Build history of the part. All positions in model axes, mm. A direction names the side the tool comes from. Round coordinates to 2 decimals unless told otherwise and drop trailing zeros. Order: outer loops, then holes, each group sorted by start corner. A loop starts at its lowest first (then second) coordinate and runs counter-clockwise, first axis right, second up. Notation, with made-up numbers: M 8,75.5 L 30,75.5 A9 cw 30,89.5 Z; hole C 53.25,29.25 d2. An arc over 180 degrees is marked long. Use CSV: the item, a comma, the result in double quotes.
from build123d import *

# Parameters (mm, degrees)
SKETCH1_W                    = 50
SKETCH1_H                    = 50
BASE_FLANGE2_DEPTH           = 3
EDGE_FLANGE1_STRIP_W         = 16
EDGE_FLANGE1_STRIP_H         = 3
EDGE_FLANGE1_STRIP_CUT_DEPTH = 50
EDGE_FLANGE1_DEPTH           = 50
EDGE_FLANGE1_PROFILE_R       = 6.25
EDGE_FLANGE1_PROFILE_R_2     = 5.5
EDGE_FLANGE1_FLAT_DEPTH      = 3
SKETCH22_R                   = 6.5
CUT_EXTRUDE1_DEPTH           = 10


# Sheet-metal steps are written as plain solids
with BuildPart() as part:
    # Sketch1 → Base-Flange2 (new body)
    with BuildSketch(Plane.XY):
        Rectangle(SKETCH1_W, SKETCH1_H)
    extrude(amount=-BASE_FLANGE2_DEPTH)

    # Edge-Flange1 strip (across the edge) → Edge-Flange1 strip cut (cut)
    with BuildSketch(Plane(origin=(25, -25, 0), x_dir=(-1, 0, 0), z_dir=(0, 1, 0))):
        with Locations((-3, -1.5)):
            Rectangle(EDGE_FLANGE1_STRIP_W, EDGE_FLANGE1_STRIP_H)
    edge_flange1_strip_cut = extrude(amount=EDGE_FLANGE1_STRIP_CUT_DEPTH, mode=Mode.SUBTRACT)

    # Edge-Flange1 bend section (across the edge) → Edge-Flange1 (add)
    with BuildSketch(Plane(origin=(25, -25, 0), x_dir=(-1, 0, 0), z_dir=(0, 1, 0))):
        with BuildLine():
            Line((0, 2), (3, 2))
            ThreePointArc((3, 2), (3.585786438, 0.585786438), (5, 0))
            Line((5, 0), (5, -3))
            ThreePointArc((5, -3), (1.464466094, -1.535533906), (0, 2))
        make_face()
    edge_flange1 = extrude(amount=EDGE_FLANGE1_DEPTH)

    # Edge-Flange1 profile (on flange) → Edge-Flange1 flat (add)
    with BuildSketch(Plane.YZ.offset(25)):
        with BuildLine():
            ThreePointArc((32.731549172, 73.12961498), (30.399526878, 85.843718314), (17.474995057, 85.635802941))
            Line((17.474995057, 85.635802941), (-17.56059029, 55.179833247))
            ThreePointArc((-17.56059029, 55.179833247), (-20.099612709, 51.779669871), (-21, 47.632737445))
            Line((-21, 47.632737445), (-21, 27.69))
            Line((-21, 27.69), (-25, 25.69))
            Line((-25, 25.69), (-25, 2))
            Line((-25, 2), (25, 2))
            Line((25, 2), (25, 25.69))
            Line((25, 25.69), (21, 27.69))
            Line((21, 27.69), (21, 52.19))
            Line((21, 52.19), (32.731549172, 73.12961498))
        make_face()
        with Locations((0, 52.19)):
            Circle(EDGE_FLANGE1_PROFILE_R, mode=Mode.SUBTRACT)
        with Locations((24.06, 78.11)):
            Circle(EDGE_FLANGE1_PROFILE_R_2, mode=Mode.SUBTRACT)
    edge_flange1_flat = extrude(amount=-EDGE_FLANGE1_FLAT_DEPTH)

    # Mirror1: Edge-Flange1 strip cut, Edge-Flange1, Edge-Flange1 flat across plane
    add(edge_flange1_strip_cut.mirror(Plane(origin=(0, 0, 0), x_dir=(0, 0, 1), z_dir=(1, 0, 0))), mode=Mode.SUBTRACT)
    add(edge_flange1.mirror(Plane(origin=(0, 0, 0), x_dir=(0, 0, 1), z_dir=(1, 0, 0))))
    add(edge_flange1_flat.mirror(Plane(origin=(0, 0, 0), x_dir=(0, 0, 1), z_dir=(1, 0, 0))))

    # Sketch22 → Cut-Extrude1 (cut)
    with BuildSketch(Plane(origin=(0, 0, -3), x_dir=(-1, 0, 0), z_dir=(0, 0, -1))):
        Circle(SKETCH22_R)
    extrude(amount=-CUT_EXTRUDE1_DEPTH, mode=Mode.SUBTRACT)


solid = part.part
(1) Cut at A-A, the plane x = 0. Give the cut face in (y, z), and give its area (3 significant figures).
Answer block:
outline,"M -25,-3 L -6.5,-3 L -6.5,0 L -25,0 Z; M 6.5,-3 L 25,-3 L 25,0 L 6.5,0 Z"
area,"111 mm²"
(2) Cut at C-C, the plane y = 22. Give the cut face in (x, z), and give its area (3 significant figures).
Answer block:
outline,"M -25,2 A5 ccw -20,-3 L 20,-3 A5 ccw 25,2 L 25,27.19 L 22,27.19 L 22,2 A2 cw 20,0 L -20,0 A2 cw -22,2 L -22,27.19 L -25,27.19 Z; M -25,53.97 L -22,53.97 L -22,73.01 L -25,73.01 Z; M -25,83.21 L -22,83.21 L -22,87.9 L -25,87.9 Z; M 22,53.97 L 25,53.97 L 25,73.01 L 22,73.01 Z; M 22,83.21 L 25,83.21 L 25,87.9 L 22,87.9 Z"
area,"446 mm²"
(3) Cut at B-B, the plane z = 10. Give the cut face in (x, y).
Answer block:
outline,"M -25,-25 L -22,-25 L -22,25 L -25,25 Z; M 22,-25 L 25,-25 L 25,25 L 22,25 Z"
(4) Two-plate mould, pull along Z, no slides. Class faces 1 (the face through (23.521, -20.075, 51.834)), 2 (the face through (-22, 4, 36)), 3 (the face through (-23.521, 23.028, 26.676)): released by +Z, released by -Z, zero draft, split by the parting line, or undercut.
Answer block:
face 1,"released by +Z"
face 2,"zero draft"
face 3,"undercut"
(5) Cut at D-D, the plane y = 2. Give the cut face in (x, z), and give its area (3 significant figures).
Answer block:
outline,"M -25,2 A5 ccw -20,-3 L -6.18,-3 L -6.18,0 L -20,0 A2 cw -22,2 L -22,46.27 L -25,46.27 Z; M -25,58.11 L -22,58.11 L -22,72.18 L -25,72.18 Z; M 6.18,-3 L 20,-3 A5 ccw 25,2 L 25,46.27 L 22,46.27 L 22,2 A2 cw 20,0 L 6.18,0 Z; M 22,58.11 L 25,58.11 L 25,72.18 L 22,72.18 Z"
area,"466 mm²"
(6) Wall check: line 1 (Y direction, x = 0, z = -1.15); line 2 (X direction, y = 10.5, z = 14); line 3 (Z direction, x = -15.5, y = -15). Give the ranges that are in metal, low to high. Write a range as from..to.
Answer block:
line 1,"y = -25..-6.5, 6.5..25"
line 2,"x = -25..-22, 22..25"
line 3,"z = -3..0"
(7) Drop flat-ended pins along their axis: pin 1 (2.5 mm diameter, centred on x = -23.5, z = 35.5, fed in from -Y); pin 2 (3.5 mm diameter, centred on x = -23, z = 44.5, fed in from +Y); pin 3 (17 mm diameter, centred on x = 0, y = 0, fed in from +Z). Give the stop position or say it passes through.
Answer block:
pin 1,"stops at y = -21"
pin 2,"stops at y = 21"
pin 3,"stops at z = 0"
(8) Tool access for faces 4 (the face through (-0.1, 25, -0.4)), 5 (the face through (23.52, 26.6, 73.23)), 6 (the face through (-21.43, -0.35, 0.6)), 7 (the face through (24, -21, 38)), 8 (the face through (-24, 21, 40)): list every direction of +Z, -Z, +X, -X, +Y, -Y with a clear straight run to the whole face (end or side of a thin tool).
Answer block:
face 4,"-Z, +X, -X, +Y"
face 5,"+X, -X"
face 6,"+Z, +Y, -Y"
face 7,"+Z, +X, -X, -Y"
face 8,"+X, -X, +Y"
